from build123d import *

# Parameters (mm, degrees)
SKETCH_1_W      = 82
SKETCH_1_H      = 60
SKETCH_1_R      = 1.1
SKETCH_1_R_2    = 1.6
SKETCH_1_W_2    = 12
SKETCH_1_H_2    = 24
EXTRUDE_1_DEPTH = 3


with BuildPart() as part:
    # 草图1 → 凸台-拉伸1 (new body)
    with BuildSketch(Plane.XY):
        with Locations((41, 30)):
            Rectangle(SKETCH_1_W, SKETCH_1_H)
        with Locations((18.5, 44)):
            Circle(SKETCH_1_R, mode=Mode.SUBTRACT)
        with Locations(Location((18.5, 16, 0), (0, 0, 180))):
            Circle(SKETCH_1_R, mode=Mode.SUBTRACT)
        with Locations((77, 8)):
            Circle(SKETCH_1_R_2, mode=Mode.SUBTRACT)
        with Locations(Location((5, 8, 0), (0, 0, 180))):
            Circle(SKETCH_1_R_2, mode=Mode.SUBTRACT)
        with Locations(Location((77, 52, 0), (0, 0, 180))):
            Circle(SKETCH_1_R_2, mode=Mode.SUBTRACT)
        with Locations((5, 52)):
            Circle(SKETCH_1_R_2, mode=Mode.SUBTRACT)
        with Locations((63.5, 16)):
            Circle(SKETCH_1_R, mode=Mode.SUBTRACT)
        with Locations(Location((63.5, 44, 0), (0, 0, 180))):
            Circle(SKETCH_1_R, mode=Mode.SUBTRACT)
        with Locations((63.5, 30)):
            Rectangle(SKETCH_1_W_2, SKETCH_1_H_2, mode=Mode.SUBTRACT)
        with Locations((18.5, 30)):
            Rectangle(SKETCH_1_W_2, SKETCH_1_H_2, mode=Mode.SUBTRACT)
    extrude(amount=EXTRUDE_1_DEPTH)


solid = part.part
Part model, mm, in its own coordinate system. A direction names the side the tool comes from. Coordinates: 2 decimals unless noted, no trailing zeros. Order: outer loops, then holes, each group sorted by start corner. A loop starts at its lowest first (then second) coordinate and runs counter-clockwise, first axis right, second up. Notation, with made-up numbers: (80.5, 46) - (90.5, 46) arc R31 cw to (90.5, 74) - close; hole circle Ø7 at (-25, 55.5). An arc over 180 degrees is marked (long way). Use CSV: the item, a comma, the result in double quotes.
Item 1: Saw through at C-C on x = 21.5. Give the cut face in (y, z).
Solved:
outline,"(0, 0) - (18, 0) - (18, 3) - (0, 3) - close; (42, 0) - (60, 0) - (60, 3) - (42, 3) - close"
Item 2: Saw through at D-D on z = 0.55. Give the number of separate pieces and of enclosed holes in the cut face, and give its area (3 significant figures).
Solved:
separate pieces,"1"
enclosed holes,"10"
area,"4,300 mm²"
Item 3: Saw through at A-A on y = 44. Give the cut face in (x, z).
Solved:
outline,"(0, 0) - (17.4, 0) - (17.4, 3) - (0, 3) - close; (19.6, 0) - (62.4, 0) - (62.4, 3) - (19.6, 3) - close; (64.6, 0) - (82, 0) - (82, 3) - (64.6, 3) - close"
Item 4: Saw through at B-B on x = 77. Give the cut face in (y, z).
Solved:
outline,"(0, 0) - (6.4, 0) - (6.4, 3) - (0, 3) - close; (9.6, 0) - (50.4, 0) - (50.4, 3) - (9.6, 3) - close; (53.6, 0) - (60, 0) - (60, 3) - (53.6, 3) - close"
Item 5: Probe probe 1 along Y at (x, z) = (63.5, 1.75); probe 2 along X at (y, z) = (26, 0.85); probe 3 along Y at (x, z) = (5, 1.55). List the from-to ranges inside material, lowest first.
Solved:
probe 1,"y = 0 to 14.9, 17.1 to 18, 42 to 42.9, 45.1 to 60"
probe 2,"x = 0 to 12.5, 24.5 to 57.5, 69.5 to 82"
probe 3,"y = 0 to 6.4, 9.6 to 50.4, 53.6 to 60"
Item 6: 3-axis set-ups, long thin cutter, end or side, ignore diameter. For faces 4 (the face through (40, 30, 3)), 5 (the face through (18, 42, 1)): which of +Z, -Z, +X, -X, +Y, -Y reach the whole face in a straight line?
Solved:
face 4,"+Z, +X, -X, +Y, -Y"
face 5,"+Z, -Z"
Item 7: Drop flat-ended pins along their axis: P1, Ø1.9, axis at x = 5, y = 52, coming from the +Z side; P2, Ø1.5, axis at y = 34, z = 2, coming from the -X side. Give the stop position or say it passes through.
Solved:
P1,"passes through"
P2,"stops at x = 0"
Item 8: Mould opens along Y. For faces 1 (the face through (12.5, 30, 1)), 2 (the face through (40, 60, 1)), 3 (the face through (82, 30, 1)) say: +Y half, -Y half, draft (parallel to the pull), parting line (faces both ways), or undercut.
Solved:
face 1,"undercut"
face 2,"+Y half"
face 3,"draft"
